Source: CAD feature listing. Evaluate the final solid. Frame: model axes, mm. Coordinates: 2 decimals unless noted, no trailing zeros. Loops run counter-clockwise (first coordinate to the right, second up) from the corner with the lowest first, then second, coordinate; pieces in that order, holes last.
Item 1: Section query D-D, the plane z = 10. State how many separate pieces and enclosed holes the cut face has, then the cut area to 3 significant figures.
Item 2: Section query B-B, the plane y = 5.25. Return the cut outline in (x, z), then the cut area to 3 significant figures.
Item 3: Section query C-C, the plane x = -41. Return the cut outline in (y, z), then the cut area to 3 significant figures.
Item 4: Pull-direction query (Z, two-part tool) for faces 1 (the flat face through (-24, 10, 0)), 2 (the flat face through (-21, 5, -16)), 3 (the cylindrical face through (-10.74, 4.93, -2.38)); classes: +Z half, -Z half, draft (parallel to the pull), parting line (faces both ways), or undercut.
Item 5: Line query: probe 1 along X at (y, z) = (7.75, 0); probe 2 along X at (y, z) = (5, 9); probe 3 along Z at (x, y) = (-44, 2). Output: solid intervals per line, ascending.
Item 6: Section query A-A, the plane z = 0. Return the cut outline in (x, y).
```python
from build123d import *

# Parameters (mm, degrees)
SKETCH_1_R      = 11
SKETCH_1_R_2    = 2.5
EXTRUDE_1_DEPTH = 10
CHAMFER_1_SIZE  = 1


with BuildPart() as part:
    # 草图1 → 凸台-拉伸1 (new body)
    with BuildSketch(Plane(origin=(0, 0, 0), x_dir=(1, 0, 0), z_dir=(0, 1, 0))):
        with BuildLine():
            Line((0, 16), (-42, 16))
            ThreePointArc((-42, 16), (-46.949747468, 13.949747468), (-49, 9))
            Line((-49, 9), (-49, -15))
            Line((-49, -15), (-48, -16))
            Line((-48, -16), (0, -16))
            ThreePointArc((0, -16), (16, 0), (0, 16))
        make_face()
        with Locations(Location((0, 0, 0), (0, 0, 270))):
            Circle(SKETCH_1_R, mode=Mode.SUBTRACT)
        with Locations(Location((-42, 9, 0), (0, 0, 270))):
            Circle(SKETCH_1_R_2, mode=Mode.SUBTRACT)
        with Locations(Location((-42, -9, 0), (0, 0, 270))):
            Circle(SKETCH_1_R_2, mode=Mode.SUBTRACT)
    extrude(amount=EXTRUDE_1_DEPTH)

    # 倒角1
    # the kernel refuses this chamfer: 1 mm, written as the material it takes off along each edge
    with BuildSketch(Plane(origin=(-50.571682988, 0, 16), x_dir=(0, 0.9996219169112968, 0.02749587661058563), z_dir=(1, 0, 0))) as chamfer_1_piece_1:
        Polygon((CHAMFER_1_SIZE * 0.999621916911, -CHAMFER_1_SIZE * 0.0274958766106), (-CHAMFER_1_SIZE * 0.0274958766106, -CHAMFER_1_SIZE * 0.999621916911), (0, 0), align=None)
    extrude(amount=50.571682988, mode=Mode.SUBTRACT)
    with BuildSketch(Plane(origin=(0, 0, 0), x_dir=(0, 0, 1), z_dir=(-1, 0, 0))) as chamfer_1_piece_2:
        Polygon((16, CHAMFER_1_SIZE), (16 - CHAMFER_1_SIZE, 0), (16, 0), align=None)
    revolve(axis=Axis((0, 0, 0), (0, 1, 0)), revolution_arc=180, mode=Mode.SUBTRACT)
    with BuildSketch(Plane(origin=(0, 0, -16), x_dir=(0, 0.9996219169112968, -0.02749587661058563), z_dir=(-1, 0, 0))) as chamfer_1_piece_3:
        Polygon((CHAMFER_1_SIZE * 0.999621916911, -CHAMFER_1_SIZE * 0.0274958766106), (-CHAMFER_1_SIZE * 0.0274958766106, -CHAMFER_1_SIZE * 0.999621916911), (0, 0), align=None)
    extrude(amount=42, mode=Mode.SUBTRACT)
    with BuildSketch(Plane(origin=(-42, 0, -9), x_dir=(0, 0, -1), z_dir=(1, 0, 0))) as chamfer_1_piece_4:
        Polygon((7, CHAMFER_1_SIZE), (7 - CHAMFER_1_SIZE, 0), (7, 0), align=None)
    revolve(axis=Axis((-42, 0, -9), (0, 1, 0)), revolution_arc=90, mode=Mode.SUBTRACT)
    with BuildSketch(Plane(origin=(-49, 0, -9), x_dir=(-0.02749587661058908, 0.9996219169112968, 0), z_dir=(0, 0, 1))) as chamfer_1_piece_5:
        Polygon((CHAMFER_1_SIZE * 0.999621916911, -CHAMFER_1_SIZE * 0.0274958766106), (-CHAMFER_1_SIZE * 0.0274958766106, -CHAMFER_1_SIZE * 0.999621916911), (0, 0), align=None)
    extrude(amount=26.571682988, mode=Mode.SUBTRACT)


solid = part.part
```
Verdict:
1. separate pieces: 3
1. enclosed holes: 0
1. area: 476 mm2
2. outline: (-49, -9) arc R7 ccw to (-42, -16) - (0, -16) arc R16 ccw to (0, 16) - (-48, 16) - (-49, 15) - close; hole circle Ø5 at (-42, -9); hole circle Ø5 at (-42, 9); hole circle Ø22 at (0, 0)
2. area: 1,540 mm2
3. outline: (0, -15) - (1, -16) - (10, -16) - (10, -11.29) - (0, -11.29) - close; (0, -6.71) - (10, -6.71) - (10, 6.71) - (0, 6.71) - close; (0, 11.29) - (10, 11.29) - (10, 16) - (1, 16) - (0, 15) - close
3. area: 227 mm2
4. face 1: draft
4. face 2: -Z half
4. face 3: undercut
5. probe 1: x = -49 to -11, 11 to 16
5. probe 2: x = -49 to -44.5, -39.5 to -6.32, 6.32 to 13.23
5. probe 3: z = -15.71 to -10.5, -7.5 to 7.5, 10.5 to 16
6. outline: (-49, 1) - (-48, 0) - (-11, 0) - (-11, 10) - (-49, 10) - close; (11, 0) - (15, 0) - (16, 1) - (16, 10) - (11, 10) - close
